from build123d import *

# Parameters (mm, degrees)
SKETCH1_W           = 54
SKETCH1_H           = 39
SKETCH1_W_2         = 10
SKETCH1_H_2         = 10
SKETCH1_R           = 2.5527
BOSS_EXTRUDE1_DEPTH = 8
SKETCH2_W           = 50.1
SKETCH2_H           = 35.1
CUT_EXTRUDE1_DEPTH  = 0.0762
CUT_EXTRUDE2_DEPTH  = 6.5
SKETCH4_R           = 1.56
CUT_EXTRUDE3_DEPTH  = 43.568023286
SKETCH5_R           = 1.79
CUT_EXTRUDE4_DEPTH  = 2.92
SKETCH6_W           = 12.25
SKETCH6_H           = 15.75
SKETCH6_W_2         = 15.75
SKETCH6_H_2         = 12.5
SKETCH6_W_3         = 5.5
SKETCH6_H_3         = 5.5
CUT_EXTRUDE5_DEPTH  = 43.337883821
CHAMFER1_SIZE       = 0.5
FILLET1_R           = 1


with BuildPart() as part:
    # Sketch1 → Boss-Extrude1 (new body)
    # profile 1 of 3: a face of its own
    with BuildSketch(Plane(origin=(0, 0, 0), x_dir=(1, 0, 0), z_dir=(0, 1, 0))):
        Rectangle(SKETCH1_W, SKETCH1_H)
    # profile 2 of 3: a face of its own
    with BuildSketch(Plane(origin=(0, 0, 0), x_dir=(1, 0, 0), z_dir=(0, 1, 0))):
        with Locations((32, 0)):
            Rectangle(SKETCH1_W_2, SKETCH1_H_2)
        with Locations(Location((32, 0, 0), (0, 0, 270))):
            Circle(SKETCH1_R, mode=Mode.SUBTRACT)
    # profile 3 of 3: a face of its own
    with BuildSketch(Plane(origin=(0, 0, 0), x_dir=(1, 0, 0), z_dir=(0, 1, 0))):
        with Locations((-32, 0)):
            Rectangle(SKETCH1_W_2, SKETCH1_H_2)
        with Locations(Location((-32, 0, 0), (0, 0, 270))):
            Circle(SKETCH1_R, mode=Mode.SUBTRACT)
    extrude(amount=BOSS_EXTRUDE1_DEPTH)

    # Sketch2 → Cut-Extrude1 (cut)
    with BuildSketch(Plane(origin=(0, 8, 0), x_dir=(1, 0, 0), z_dir=(0, 1, 0))):
        Rectangle(SKETCH2_W, SKETCH2_H)
    extrude(amount=-CUT_EXTRUDE1_DEPTH, mode=Mode.SUBTRACT)

    # Sketch3 → Cut-Extrude2 (cut)
    with BuildSketch(Plane(origin=(0, 7.9238, 0), x_dir=(1, 0, 0), z_dir=(0, 1, 0))):
        with BuildLine():
            Line((-3.79, 14.5), (-3.79, 17.55))
            Line((-3.79, 17.55), (-25.05, 17.55))
            Line((-25.05, 17.55), (-25.05, -10.71))
            Line((-25.05, -10.71), (-22, -10.71))
            ThreePointArc((-22, -10.71), (-19.320065299, -11.820065299), (-18.21, -14.5))
            Line((-18.21, -14.5), (-18.21, -17.55))
            Line((-18.21, -17.55), (18.21, -17.55))
            Line((18.21, -17.55), (18.21, -14.5))
            ThreePointArc((18.21, -14.5), (19.320065299, -11.820065299), (22, -10.71))
            Line((22, -10.71), (25.05, -10.71))
            Line((25.05, -10.71), (25.05, 17.55))
            Line((25.05, 17.55), (3.79, 17.55))
            Line((3.79, 17.55), (3.79, 14.5))
            ThreePointArc((3.79, 14.5), (0, 10.71), (-3.79, 14.5))
        make_face()
    extrude(amount=-CUT_EXTRUDE2_DEPTH, mode=Mode.SUBTRACT)

    # Sketch4 → Cut-Extrude3 (cut, through all)
    with BuildSketch(Plane(origin=(0, 7.9238, 0), x_dir=(1, 0, 0), z_dir=(0, 1, 0))):
        with Locations(Location((0, 14.5, 0), (0, 0, 270))):
            Circle(SKETCH4_R)
        with Locations(Location((-22, -14.5, 0), (0, 0, 270))):
            Circle(SKETCH4_R)
        with Locations(Location((22, -14.5, 0), (0, 0, 90))):
            Circle(SKETCH4_R)
    extrude(amount=-CUT_EXTRUDE3_DEPTH, mode=Mode.SUBTRACT)

    # Sketch5 → Cut-Extrude4 (cut)
    with BuildSketch(Plane(origin=(0, 7.9238, 0), x_dir=(1, 0, 0), z_dir=(0, 1, 0))):
        with Locations(Location((0, 14.5, 0), (0, 0, 270))):
            Circle(SKETCH5_R)
        with Locations(Location((-22, -14.5, 0), (0, 0, 270))):
            Circle(SKETCH5_R)
        with Locations(Location((22, -14.5, 0), (0, 0, 90))):
            Circle(SKETCH5_R)
    extrude(amount=-CUT_EXTRUDE4_DEPTH, mode=Mode.SUBTRACT)

    # Sketch6 → Cut-Extrude5 (cut, through all)
    with BuildSketch(Plane(origin=(0, 1.4238, 0), x_dir=(1, 0, 0), z_dir=(0, 1, 0))):
        with Locations((17.975, 6.255)):
            Rectangle(SKETCH6_W, SKETCH6_H)
        with Locations((7.975, -10.15)):
            Rectangle(SKETCH6_W_2, SKETCH6_H_2)
        with Locations((-17.975, 6.255)):
            Rectangle(SKETCH6_W, SKETCH6_H)
        with Locations((-8.4, -10.15)):
            Rectangle(SKETCH6_W_2, SKETCH6_H_2)
        with Locations((-8.45, 13.8)):
            Rectangle(SKETCH6_W_3, SKETCH6_H_3)
    extrude(amount=-CUT_EXTRUDE5_DEPTH, mode=Mode.SUBTRACT)

    # Chamfer1
    chamfer1_edges = [part.edges().sort_by_distance(p)[0] for p in [
        (-27, 0, 12.25),
        (-32, 0, 5),
        (-37, 0, 0),
        (-32, 0, -5),
        (-27, 0, -12.25),
        (0, 0, -19.5),
        (27, 0, -12.25),
        (32, 0, -5),
        (37, 0, 0),
        (32, 0, 5),
        (27, 0, 12.25),
        (0, 0, 19.5),
    ]]
    chamfer(chamfer1_edges, length=CHAMFER1_SIZE)

    # Fillet1
    fillet1_edges = [part.edges().sort_by_distance(p)[0] for p in [
        (-27, 4.25, 19.5),
        (-27, 4.25, 5),
        (-37, 4.25, 5),
        (-37, 4.25, -5),
        (-27, 4.25, -5),
        (-27, 4.25, -19.5),
        (27, 4.25, -19.5),
        (27, 4.25, -5),
        (37, 4.25, -5),
        (37, 4.25, 5),
        (27, 4.25, 5),
        (27, 4.25, 19.5),
    ]]
    fillet(fillet1_edges, radius=FILLET1_R)


solid = part.part
Input: part model. Units: mm. Frame: model coordinates. A direction names the side the tool comes from. Give positions to 0.01 mm unless a question says otherwise; leave off trailing zeros. Write each loop counter-clockwise with the first axis right and the second up, starting at its lowest first coordinate (ties: lowest second). Pieces come first, ordered by that corner, then holes. Notation, with made-up numbers: M 87,26.25 L 125,26.25 A26 ccw 125,40.25 Z; hole C 55.25,-34.75 d2. An arc over 180 degrees is marked long. Write item = value, one per line. Start each with the question number.
1) Cut plane D-D on z = 12. Return the cut outline in (x, y) (3 decimals), then the cut area to 3 significant figures.
2) Cut plane C-C on x = 15. Return the cut outline in (y, z).
3) Cut plane B-B on z = 0. Return the cut outline in (x, y), then the cut area to 3 significant figures.
4) Cut plane A-A on x = 7. Return the cut outline in (y, z).
5) Reachability of faces 5 (the flat face through (3.79, 5, -16)), 6 (the flat face through (0, 4, -19.5)), 7 (the flat face through (-9, 1, 16.4)) from +Z, -Z, +X, -X, +Y, -Y: full face, straight path, thin tool, end or side. Return the list, or none.
6) First-contact query: pin 1 Ø4 at (x, z) = (-29.5, -10) entering from +Y; pin 2 Ø1.1 at (y, z) = (0.5, -13.5) entering from -X; pin 3 Ø2 at (x, z) = (24.5, -10.5) entering from +Y; pin 4 Ø2 at (x, z) = (22, 13.5) entering from +Y. Flat tips, straight axial feed; report the tip coordinate or a pass-through.
7) Draft query along X for faces 1 (the flat face through (37, 4, 0)), 2 (the flat face through (-37, 4, 0)), 3 (the flat face through (24, 5, 10.71)), 4 (the flat face through (0, 4, 19.5)). Return one class per face: +X half, -X half, draft (parallel to the pull), parting line (faces both ways), or undercut.
8) Material intervals for line 1 along X through (y, z) = (2.5, 0); line 2 along X through (y, z) = (2.85, 14.5); line 3 along Z through (x, y) = (22, 2.75), sorted ascending. Write a range as [from, to].
Solved:
q1.outline = M -27,0.5 L -26.5,0 L -16.275,0 L -16.275,1.424 L -19.151,1.424 L -19.151,7.924 L -25.05,7.924 L -25.05,8 L -27,8 Z; M -0.525,0 L 0.1,0 L 0.1,1.424 L -0.525,1.424 Z; M 15.85,0 L 26.5,0 L 27,0.5 L 27,8 L 25.05,8 L 25.05,7.924 L 19.151,7.924 L 19.151,1.424 L 15.85,1.424 Z
q1.area = 134 mm2
q2.outline = M 0,-19 L 0.5,-19.5 L 8,-19.5 L 8,-17.55 L 1.42,-17.55 L 1.42,-14.13 L 0,-14.13 Z; M 0,1.62 L 1.42,1.62 L 1.42,3.9 L 0,3.9 Z; M 0,16.4 L 1.42,16.4 L 1.42,17.55 L 8,17.55 L 8,19.5 L 0.5,19.5 L 0,19 Z
q3.outline = M -37,0.5 L -36.5,0 L -34.55,0 L -34.55,8 L -37,8 Z; M -29.45,0 L -24.1,0 L -24.1,1.42 L -25.05,1.42 L -25.05,8 L -29.45,8 Z; M -11.85,0 L 11.85,0 L 11.85,1.42 L -11.85,1.42 Z; M 24.1,0 L 29.45,0 L 29.45,8 L 25.05,8 L 25.05,1.42 L 24.1,1.42 Z; M 34.55,0 L 36.5,0 L 37,0.5 L 37,8 L 34.55,8 Z
q3.area = 146 mm2
q4.outline = M 0,-19 L 0.5,-19.5 L 8,-19.5 L 8,-17.55 L 1.42,-17.55 L 1.42,3.9 L 0,3.9 Z; M 0,16.4 L 1.42,16.4 L 1.42,17.55 L 8,17.55 L 8,19.5 L 0.5,19.5 L 0,19 Z
q5.face_5 = +Y
q5.face_6 = -Z, +X, -X, +Y, -Y
q5.face_7 = +Y, -Y
q6.pin_1 = through
q6.pin_2 = -27
q6.pin_3 = 8
q6.pin_4 = 7.92
q7.face_1 = +X half
q7.face_2 = -X half
q7.face_3 = undercut
q7.face_4 = draft
q8.line_1 = [-37, -34.55], [-29.45, -25.05], [25.05, 29.45], [34.55, 37]
q8.line_2 = [-27, -23.56], [-20.44, -18.21], [18.21, 20.44], [23.56, 27]
q8.line_3 = [-19.5, -17.55], [10.71, 12.94], [16.06, 19.5]
